CAD build for the part. Positions are in the model's coordinates, mm. Round coordinates to 2 decimals unless told otherwise and drop trailing zeros. Order: outer loops, then holes, each group sorted by start corner. A loop starts at its lowest first (then second) coordinate and runs counter-clockwise, first axis right, second up. Notation, with made-up numbers: (-1, 68.5) - (27, 68.5) arc R27 ccw to (27, 92.5) - close; hole circle Ø11 at (3.5, -0.5). An arc over 180 degrees is marked (long way). Write item = value, one per line.
from build123d import *

# Parameters (mm, degrees)
CYLINDER005_R     = 2
CYLINDER005_DEPTH = 10
CYLINDER004_R     = 2
CYLINDER004_DEPTH = 10
CYLINDER002_R     = 2
CYLINDER002_DEPTH = 10
CYLINDER003_R     = 2
CYLINDER003_DEPTH = 10
CYLINDER_R        = 2
CYLINDER_DEPTH    = 10
CYLINDER001_R     = 2
CYLINDER001_DEPTH = 10
BOX_W             = 25
BOX_H             = 15
BOX_DEPTH         = 10


with BuildPart() as cilindro005:
    # Cylinder005 → Cylinder005 (new body)
    with BuildSketch(Plane(origin=(19, 11, 0), x_dir=(1, 0, 0), z_dir=(0, 0, 1))):
        Circle(CYLINDER005_R)
    extrude(amount=CYLINDER005_DEPTH)


with BuildPart() as fusion:
    # Cylinder004 → Cylinder004 (new body)
    with BuildSketch(Plane(origin=(12, 11, 0), x_dir=(1, 0, 0), z_dir=(0, 0, 1))):
        Circle(CYLINDER004_R)
    extrude(amount=CYLINDER004_DEPTH)

    # Fusion: union Cilindro005
    add(cilindro005.part)


with BuildPart() as cilindro002:
    # Cylinder002 → Cylinder002 (new body)
    with BuildSketch(Plane(origin=(19, 5, 0), x_dir=(1, 0, 0), z_dir=(0, 0, 1))):
        Circle(CYLINDER002_R)
    extrude(amount=CYLINDER002_DEPTH)


with BuildPart() as fusion001:
    # Cylinder003 → Cylinder003 (new body)
    with BuildSketch(Plane(origin=(5, 11, 0), x_dir=(1, 0, 0), z_dir=(0, 0, 1))):
        Circle(CYLINDER003_R)
    extrude(amount=CYLINDER003_DEPTH)

    # Fusion001: union Cilindro002
    add(cilindro002.part)


with BuildPart() as cilindro:
    # Cylinder → Cylinder (new body)
    with BuildSketch(Plane(origin=(5, 5, 0), x_dir=(1, 0, 0), z_dir=(0, 0, 1))):
        Circle(CYLINDER_R)
    extrude(amount=CYLINDER_DEPTH)


with BuildPart() as agujeros:
    # Cylinder001 → Cylinder001 (new body)
    with BuildSketch(Plane(origin=(12, 5, 0), x_dir=(1, 0, 0), z_dir=(0, 0, 1))):
        Circle(CYLINDER001_R)
    extrude(amount=CYLINDER001_DEPTH)

    # Fusion002: union Cilindro
    add(cilindro.part)

    # Fusion003: union Fusion, Fusion001
    add(fusion.part)
    add(fusion001.part)


with BuildPart() as obj1:
    # Box → Box (new body)
    with BuildSketch(Plane.XY):
        with Locations((12.5, 7.5)):
            Rectangle(BOX_W, BOX_H)
    extrude(amount=BOX_DEPTH)

    # Cut: cut agujeros
    add(agujeros.part, mode=Mode.SUBTRACT)


solid = obj1.part
(1) Pull direction Y, two halves, no side cores. Call faces 1 (the cylindrical face through (17, 5, 5)), 2 (the flat face through (12, 0, 5)), 3 (the flat face through (25, 7, 5)): released by +Y, released by -Y, zero draft, split by the parting line, or undercut.
Solved:
face_1 = undercut
face_2 = released by -Y
face_3 = zero draft
(2) Band-saw the part on C-C on z = 4. List the corners of the cut face in (x, y).
Solved:
outline = (0, 0) - (25, 0) - (25, 15) - (0, 15) - close; hole circle Ø4 at (5, 5); hole circle Ø4 at (5, 11); hole circle Ø4 at (12, 5); hole circle Ø4 at (12, 11); hole circle Ø4 at (19, 5); hole circle Ø4 at (19, 11)
(3) Probe line 1 along Y through (x, z) = (5, 4); line 2 along X through (y, z) = (9.25, 7); line 3 along Y through (x, z) = (13.75, 8.25). List the from-to ranges inside material, lowest first.
Solved:
line_1 = 0 to 3, 7 to 9, 13 to 15
line_2 = 0 to 4.03, 5.97 to 11.03, 12.97 to 18.03, 19.97 to 25
line_3 = 0 to 4.03, 5.97 to 10.03, 11.97 to 15
(4) Band-saw the part on A-A on y = 5. List the corners of the cut face in (x, z).
Solved:
outline = (0, 0) - (3, 0) - (3, 10) - (0, 10) - close; (7, 0) - (10, 0) - (10, 10) - (7, 10) - close; (14, 0) - (17, 0) - (17, 10) - (14, 10) - close; (21, 0) - (25, 0) - (25, 10) - (21, 10) - close
(5) Drop a flat-ended pin along its axis: pin 1 (3.5 mm diameter, centred on x = 19, y = 5, fed in from +Z). Give the stop position or say it passes through.
Solved:
pin_1 = through
(6) Band-saw the part on D-D on x = 18.25. List the corners of the cut face in (y, z).
Solved:
outline = (0, 0) - (3.15, 0) - (3.15, 10) - (0, 10) - close; (6.85, 0) - (9.15, 0) - (9.15, 10) - (6.85, 10) - close; (12.85, 0) - (15, 0) - (15, 10) - (12.85, 10) - close
(7) Band-saw the part on B-B on x = 12. List the corners of the cut face in (y, z), plus the area to 3 significant figures.
Solved:
outline = (0, 0) - (3, 0) - (3, 10) - (0, 10) - close; (7, 0) - (9, 0) - (9, 10) - (7, 10) - close; (13, 0) - (15, 0) - (15, 10) - (13, 10) - close
area = 70.0 mm²
